```python
from build123d import *

# Parameters (mm, degrees)
SKETCH1_W           = 30
SKETCH1_H           = 10
BOSS_EXTRUDE1_DEPTH = 5


with BuildPart() as part:
    # Sketch1 → Boss-Extrude1 (new body)
    with BuildSketch(Plane(origin=(0, 0, 0), x_dir=(1, 0, 0), z_dir=(0, 1, 0))):
        Rectangle(SKETCH1_W, SKETCH1_H)
        with BuildLine():
            ThreePointArc((11.6, 1.360147051), (7.9, 0), (11.6, -1.360147051))
            Line((11.6, -1.360147051), (11.6, 1.360147051))
        make_face(mode=Mode.SUBTRACT)
        with BuildLine():
            ThreePointArc((6.575, 1.350925609), (2.925, 0), (6.575, -1.350925609))
            Line((6.575, -1.350925609), (6.575, 1.350925609))
        make_face(mode=Mode.SUBTRACT)
        with BuildLine():
            ThreePointArc((1.55, 1.341640786), (-2.05, 0), (1.55, -1.341640786))
            Line((1.55, -1.341640786), (1.55, 1.341640786))
        make_face(mode=Mode.SUBTRACT)
        with BuildLine():
            ThreePointArc((-3.475, 1.332291259), (-7.025, 0), (-3.475, -1.332291259))
            Line((-3.475, -1.332291259), (-3.475, 1.332291259))
        make_face(mode=Mode.SUBTRACT)
        with BuildLine():
            ThreePointArc((-8.5, 1.322875656), (-12, 0), (-8.5, -1.322875656))
            Line((-8.5, -1.322875656), (-8.5, 1.322875656))
        make_face(mode=Mode.SUBTRACT)
    extrude(amount=-BOSS_EXTRUDE1_DEPTH)


solid = part.part
```
Geometry check sheet. Reference: the model listing, model coordinates, mm. A direction names the side the tool comes from. Coordinates: 2 decimals unless noted, no trailing zeros. Write each loop counter-clockwise with the first axis right and the second up, starting at its lowest first coordinate (ties: lowest second). Pieces come first, ordered by that corner, then holes. Notation, with made-up numbers: (12, 44.25) -> (70, 44.25) arc R17 ccw to (70, 74.25) -> close; hole circle Ø2 at (84, 20.25). An arc over 180 degrees is marked (long way). Use CSV: the item, a comma, the result in double quotes. Start each with the question number.
Item 1: Mould release check, pull along X, two halves, no side actions. Record for faces 3 (the flat face through (15, -2, 0)), 4 (the flat face through (-15, -2, 0)), 5 (the flat face through (-3.475, -2, 0)), 6 (the flat face through (-0.2, -5, 2.2)): released by +X, released by -X, zero draft, split by the parting line, or undercut.
Item 2: Cross-section at C-C, the plane x = -10. Record the cut outline in (y, z), plus the area to 3 significant figures.
Item 3: Set-up check for faces 1 (the flat face through (0, -2, -5)), 2 (the flat face through (6.575, -2, 0)): record each of +Z, -Z, +X, -X, +Y, -Y from which the full face is reachable in a straight line by a thin tool's end or side.
Item 4: Cross-section at B-B, the plane y = -1.9. Record the cut outline in (x, z) (3 decimals), plus the area to 3 significant figures.
Item 5: Cross-section at A-A, the plane x = -5. Record the cut outline in (y, z) (3 decimals).
Item 6: Thickness scan on line 1 (Z direction, x = 0, y = -1.75); line 2 (X direction, y = -4.7, z = -1.75); line 3 (X direction, y = -3.8, z = 1) (3 decimals). Record the ranges inside material, lowest first.
Answers:
1,face 3,"released by +X"
1,face 4,"released by -X"
1,face 5,"undercut"
1,face 6,"zero draft"
2,outline,"(-5, -5) -> (0, -5) -> (0, -2) -> (-5, -2) -> close; (-5, 2) -> (0, 2) -> (0, 5) -> (-5, 5) -> close"
2,area,"30.0 mm^2"
3,face 1,"-Z, +X, -X, +Y, -Y"
3,face 2,"+Y, -Y"
4,outline,"(-15, -5) -> (15, -5) -> (15, 5) -> (-15, 5) -> close; hole (-8.5, -1.323) -> (-8.5, 1.323) arc R2 ccw (long way) to start; hole (-3.475, -1.332) -> (-3.475, 1.332) arc R2.025 ccw (long way) to start; hole (1.55, -1.342) -> (1.55, 1.342) arc R2.05 ccw (long way) to start; hole (6.575, -1.351) -> (6.575, 1.351) arc R2.075 ccw (long way) to start; hole (11.6, -1.36) -> (11.6, 1.36) arc R2.1 ccw (long way) to start"
4,area,"239 mm^2"
5,outline,"(-5, -5) -> (0, -5) -> (0, -2.025) -> (-5, -2.025) -> close; (-5, 2.025) -> (0, 2.025) -> (0, 5) -> (-5, 5) -> close"
6,line 1,"-5 to -2.05, 2.05 to 5"
6,line 2,"-15 to -10.97, -9.03 to -6.02, -3.98 to -1.07, 1.07 to 3.89, 6.11 to 8.84, 11.16 to 15"
6,line 3,"-15 to -11.732, -8.5 to -6.761, -3.475 to -1.79, 1.55 to 3.182, 6.575 to 8.153, 11.6 to 15"
